Here's how the part is built. I have some questions about the finished solid (model axes, mm). A direction names the side the tool comes from. Round coordinates to 2 decimals unless told otherwise and drop trailing zeros. Loops run counter-clockwise (first coordinate to the right, second up) from the corner with the lowest first, then second, coordinate; pieces in that order, holes last. Notation, with made-up numbers: M 4,67 L 44,67 A11 cw 44,86 Z; hole C 44,42.5 d5. An arc over 180 degrees is marked long. Answer as a JSON object with one key per item and string values.
from build123d import *

# Parameters (mm, degrees)
F0_R     = 25
F1_DEPTH = 16
F2_R     = 10
F3_DEPTH = 20
F4_R     = 10
F5_SIZE  = 2
F7_D     = 6.6
F7_DEPTH = 13
F7_TIP   = 1.9828400428


with BuildPart() as f1:
    # F0 (on Front) → F1 (new body)
    with BuildSketch(Plane.XZ):
        Circle(F0_R)
    extrude(amount=F1_DEPTH)

    # F2 (on face) → F3 (join)
    with BuildSketch(Plane.XZ.offset(16)):
        Circle(F2_R)
    extrude(amount=F3_DEPTH)

    # F4
    f4_edges = [f1.edges().sort_by_distance(p)[0] for p in [
        (-25, 0, 0),
    ]]
    fillet(f4_edges, radius=F4_R)

    # F5
    f5_edges = [f1.edges().sort_by_distance(p)[0] for p in [
        (-25, -16, 0),
    ]]
    chamfer(f5_edges, length=F5_SIZE)

    # F7
    with Locations(Plane.XZ.offset(36)):
        with Locations((0, 0)):
            Hole(F7_D / 2, depth=F7_DEPTH)
            with Locations((0, 0, -(F7_DEPTH + F7_TIP / 2))):  # 118° drill point
                Cone(0, F7_D / 2, F7_TIP, mode=Mode.SUBTRACT)


solid = f1.part
Item 1: For faces 1 (the face through (0, 0, 0)), 2 (the face through (10, -16, -5)), which set-ups out of +Z, -Z, +X, -X, +Y, -Y let a thin tool reach every point of the face, with its end or its side?
Solution:
{"face 1": "+Z, -Z, +X, -X, +Y", "face 2": "-Y"}
Item 2: For P1, Ø1.5, axis at x = -6.5, z = 17, coming from the -Y side; P2, Ø6, axis at x = -11.5, y = -23.5, coming from the -Z side; P3, Ø3, axis at y = -30, z = 6.5, coming from the +X side, each with a flat end and sliding along its axis, tell me the tip position at first contact or that it passes through.
Solution:
{"P1": "stops at y = -16", "P2": "stops at z = -5.27", "P3": "stops at x = 8.66"}
Item 3: I want a section at B-B on y = -25. List the corners of the cut face in (x, z) for me, plus the area to 3 significant figures.
Solution:
{"outline": "C 0,0 d20; hole C 0,0 d6.6", "area": "280 mm2"}
Item 4: I want a section at C-C on y = -4. List the corners of the cut face in (x, z) for me.
Solution:
{"outline": "C 0,0 d46"}
Item 5: If I drill on L1, parallel to Z at x = 0, y = -28.25; L2, parallel to Y at x = -8.5, z = 7; L3, parallel to Z at x = 0, y = -17, over which ranges is the centre line in solid material (lowest first)? Write a range as from..to.
Solution:
{"L1": "z = -10..-3.3, 3.3..10", "L2": "y = -16..0", "L3": "z = -10..10"}
Item 6: We'd pull the mould along X, two halves only. Please class faces 3 (the face through (0.53, -21.36, -0.22)), 4 (the face through (4, -36, 0)), 5 (the face through (23.846, -11.972, 7.509)): +X half, -X half, draft (parallel to the pull), parting line (faces both ways), or undercut.
Solution:
{"face 3": "undercut", "face 4": "draft", "face 5": "parting line"}
Item 7: I want a section at A-A on y = -20. List the corners of the cut face in (x, z) for me.
Solution:
{"outline": "C 0,0 d20"}
